Can you work these out from the model? Positions are in its coordinate system, mm. A direction names the side the tool comes from. Round coordinates to 2 decimals unless told otherwise and drop trailing zeros. Order: outer loops, then holes, each group sorted by start corner. A loop starts at its lowest first (then second) coordinate and runs counter-clockwise, first axis right, second up. Notation, with made-up numbers: M 12,-10 L 65,-10 A12 ccw 65,-1 Z; hole C -11.5,32.5 d3. An arc over 180 degrees is marked long. Answer as a JSON object with one key per item and string values. Group by question number.
from build123d import *

# Parameters (mm, degrees)
SKETCH_R     = 4.5
SKETCH_R_2   = 1.2
PAD_DEPTH    = 4
SKETCH001_W  = 10
SKETCH001_H  = 10
POCKET_DEPTH = 3


with BuildPart() as part:
    # Sketch → Pad (new body)
    with BuildSketch(Plane.XY):
        Polygon((0, 0), (33.5, 0), (33.5, 4), (37.75, 8.25), (41.75, 8.25), (41.75, 41.75), (37.75, 41.75), (33.5, 46), (33.5, 50), (0, 50), (0, 46), (-4.25, 41.75), (-8.25, 41.75), (-8.25, 8.25), (-4.25, 8.25), (0, 4), align=None)
        with Locations((16.75, 25)):
            Circle(SKETCH_R, mode=Mode.SUBTRACT)
        with Locations((-1.25, 34.75)):
            Circle(SKETCH_R_2, mode=Mode.SUBTRACT)
        with Locations((-1.25, 14.75)):
            Circle(SKETCH_R_2, mode=Mode.SUBTRACT)
        with Locations((34.75, 34.75)):
            Circle(SKETCH_R_2, mode=Mode.SUBTRACT)
        with Locations((34.75, 14.75)):
            Circle(SKETCH_R_2, mode=Mode.SUBTRACT)
    extrude(amount=PAD_DEPTH)

    # Sketch001 → Pocket (cut)
    with BuildSketch(Plane.XY):
        with Locations((16.75, 25)):
            Rectangle(SKETCH001_W, SKETCH001_H)
    extrude(amount=POCKET_DEPTH, mode=Mode.SUBTRACT)


solid = part.part
Item 1: I'm going to push flat-ended pins straight in: pin 1 Ø2 at (x, z) = (-7, 2.5) entering from -Y; pin 2 Ø1.4 at (x, y) = (-1.25, 34.75) entering from -Z; pin 3 Ø3 at (x, y) = (34.75, 34.75) entering from +Z; pin 4 Ø2 at (y, z) = (47.5, 1.5) entering from +X. Where does each tip first touch, or does it pass through?
Item 2: Suppose I cut it at C-C, the plane y = 25. Write out the boundary of the cut face in (x, z), and give its area (3 significant figures).
Item 3: On a 3-axis mill with a long thin cutter (end or side, diameter ignored), from which of +Z, -Z, +X, -X, +Y, -Y can I reach the whole of each face in a straight line? I mean faces 1 (the face through (11.75, 25, 1)), 2 (the face through (-6, 41.75, 2)), 3 (the face through (0, 2, 2)). Say none if no direction works.
Item 4: I need wall thicknesses on line 1 (X direction, y = 25, z = 3.35); line 2 (Y direction, x = 16.75, z = 3.25); line 3 (X direction, y = 25, z = 2.15). Which ranges of each line are inside material? Lowest first, please.
Item 5: Suppose I cut it at B-B, the plane x = 16.75. Write out the boundary of the cut face in (y, z).
Item 6: Suppose I cut it at A-A, the plane y = 14.75. Write out the boundary of the cut face in (x, z).
Item 7: If we mould it in two halves opening along X, with no side actions, what happens to faces 4 (the face through (0, 48, 2)), 5 (the face through (13.43, 28.04, 3.49)), 6 (the face through (17, 30, 1)), 7 (the face through (40, 8.25, 2))? For each: +X half, -X half, draft (parallel to the pull), parting line (faces both ways), or undercut.
Item 8: Suppose I cut it at D-D, the plane x = 34.75. Write out the boundary of the cut face in (y, z), and give its area (3 significant figures).
Computed:
{
 "1": {"pin 1": "stops at y = 8.25", "pin 2": "passes through", "pin 3": "stops at z = 4", "pin 4": "stops at x = 33.5"},
 "2": {"outline": "M -8.25,0 L 11.75,0 L 11.75,3 L 12.25,3 L 12.25,4 L -8.25,4 Z; M 21.25,3 L 21.75,3 L 21.75,0 L 41.75,0 L 41.75,4 L 21.25,4 Z", "area": "161 mm^2"},
 "3": {"face 1": "-Z", "face 2": "+Z, -Z, -X, +Y", "face 3": "+Z, -Z, -X, -Y"},
 "4": {"line 1": "x = -8.25 to 12.25, 21.25 to 41.75", "line 2": "y = 0 to 20.5, 29.5 to 50", "line 3": "x = -8.25 to 11.75, 21.75 to 41.75"},
 "5": {"outline": "M 0,0 L 20,0 L 20,3 L 20.5,3 L 20.5,4 L 0,4 Z; M 29.5,3 L 30,3 L 30,0 L 50,0 L 50,4 L 29.5,4 Z"},
 "6": {"outline": "M -8.25,0 L -2.45,0 L -2.45,4 L -8.25,4 Z; M -0.05,0 L 33.55,0 L 33.55,4 L -0.05,4 Z; M 35.95,0 L 41.75,0 L 41.75,4 L 35.95,4 Z"},
 "7": {"face 4": "-X half", "face 5": "undercut", "face 6": "undercut", "face 7": "draft"},
 "8": {"outline": "M 5.25,0 L 13.55,0 L 13.55,4 L 5.25,4 Z; M 15.95,0 L 33.55,0 L 33.55,4 L 15.95,4 Z; M 35.95,0 L 44.75,0 L 44.75,4 L 35.95,4 Z", "area": "139 mm^2"}
}
